```python
from build123d import *

# Parameters (mm, degrees)
ESBO_O1_W                = 700
ESBO_O1_H                = 210
RESSALTO_EXTRUS_O1_DEPTH = 2.5
RESSALTO_EXTRUS_O2_DEPTH = 150
CORTE_EXTRUS_O3_REACH    = 212
ESBO_O3_W                = 695
ESBO_O3_H                = 120
RESSALTO_EXTRUS_O5_DEPTH = 9.58
ESBO_O7_W                = 2.5
ESBO_O7_H                = 217.08
RESSALTO_EXTRUS_O6_DEPTH = 100
ESBO_O9_W                = 2.5
ESBO_O9_H                = 9.6
CORTE_EXTRUS_O4_DEPTH    = 9.5
ESBO_O10_R               = 4.5
CORTE_EXTRUS_O5_DEPTH    = 3
ESBO_O11_W               = 700
ESBO_O11_H               = 125
ESBO_O11_W_2             = 695
ESBO_O11_H_2             = 120
RESSALTO_EXTRUS_O7_DEPTH = 50
ESBO_O12_W               = 700
ESBO_O12_H               = 125
RESSALTO_EXTRUS_O8_DEPTH = 2.5


with BuildPart() as part:
    # Esboço1 → Ressalto-extrusão1 (new body)
    with BuildSketch(Plane.XY):
        Rectangle(ESBO_O1_W, ESBO_O1_H)
    extrude(amount=RESSALTO_EXTRUS_O1_DEPTH)

    # Esboço2 → Ressalto-extrusão2 (add)
    with BuildSketch(Plane.XY.offset(2.5)):
        Polygon((-347.5, 102.5), (-347.5, -105), (-350, -105), (-350, 105), (350, 105), (350, -105), (347.5, -105), (347.5, 102.5), align=None)
    extrude(amount=RESSALTO_EXTRUS_O2_DEPTH)

    # Esboço3 → Corte-extrusão3 (cut, up to next)
    with BuildSketch(Plane(origin=(0, 105, 0), x_dir=(1, 0, 0), z_dir=(0, 1, 0)), mode=Mode.PRIVATE) as corte_extrus_o3_sk1:
        with Locations((0, -62.5)):
            Rectangle(ESBO_O3_W, ESBO_O3_H)
    corte_extrus_o3_tool1 = extrude(corte_extrus_o3_sk1.sketch, amount=-CORTE_EXTRUS_O3_REACH, mode=Mode.PRIVATE) & part.part
    add(corte_extrus_o3_tool1.solids().sort_by_distance((0, 105, 62.5))[0], mode=Mode.SUBTRACT)

    # Esboço6 → Ressalto-extrusão5 (add)
    with BuildSketch(Plane.XZ.offset(105)):
        Polygon((350, 0), (350, 152.5), (347.5, 152.5), (347.5, 2.5), (-347.5, 2.5), (-347.5, 152.5), (-350, 152.5), (-350, 0), align=None)
    extrude(amount=RESSALTO_EXTRUS_O5_DEPTH)

    # Esboço7 → Ressalto-extrusão6 (add)
    with BuildSketch(Plane.ZY.offset(-347.5)):
        with Locations((151.25, -6.04)):
            Rectangle(ESBO_O7_W, ESBO_O7_H)
    ressalto_extrus_o6 = extrude(amount=RESSALTO_EXTRUS_O6_DEPTH)

    # Espelhar1: Ressalto-extrusão6 across plane
    add(ressalto_extrus_o6.mirror(Plane(origin=(0, 0, 0), x_dir=(0, 0, 1), z_dir=(1, 0, 0))))

    # Esboço9 → Corte-extrusão4 (cut)
    with BuildSketch(Plane.XY.offset(152.5)):
        with Locations((-248.75, -109.78)):
            Rectangle(ESBO_O9_W, ESBO_O9_H)
        with Locations((248.75, -109.78)):
            Rectangle(ESBO_O9_W, ESBO_O9_H)
    extrude(amount=-CORTE_EXTRUS_O4_DEPTH, mode=Mode.SUBTRACT)

    # Esboço10 → Corte-extrusão5 (cut)
    with BuildSketch(Plane(origin=(0, 105, 0), x_dir=(1, 0, 0), z_dir=(0, 1, 0))):
        with Locations((-230, -142.29)):
            Circle(ESBO_O10_R)
        with Locations((-115, -142.29)):
            Circle(ESBO_O10_R)
        with Locations((0, -142.29)):
            Circle(ESBO_O10_R)
        with Locations((115, -142.29)):
            Circle(ESBO_O10_R)
        with Locations((230, -142.29)):
            Circle(ESBO_O10_R)
    extrude(amount=-CORTE_EXTRUS_O5_DEPTH, mode=Mode.SUBTRACT)

    # Esboço11 → Ressalto-extrusão7 (add)
    with BuildSketch(Plane(origin=(0, 105, 0), x_dir=(1, 0, 0), z_dir=(0, 1, 0))):
        with Locations((0, -62.5)):
            Rectangle(ESBO_O11_W, ESBO_O11_H)
        with Locations((0, -62.5)):
            Rectangle(ESBO_O11_W_2, ESBO_O11_H_2, mode=Mode.SUBTRACT)
    extrude(amount=RESSALTO_EXTRUS_O7_DEPTH)

    # Esboço12 → Ressalto-extrusão8 (add)
    with BuildSketch(Plane(origin=(0, 155, 0), x_dir=(1, 0, 0), z_dir=(0, 1, 0))):
        with Locations((0, -62.5)):
            Rectangle(ESBO_O12_W, ESBO_O12_H)
    extrude(amount=RESSALTO_EXTRUS_O8_DEPTH)


solid = part.part
```
Can you work these out from the model? Positions are in its coordinate system, mm. A direction names the side the tool comes from. Coordinates: 2 decimals unless noted, no trailing zeros. Write each loop counter-clockwise with the first axis right and the second up, starting at its lowest first coordinate (ties: lowest second). Pieces come first, ordered by that corner, then holes. Notation, with made-up numbers: M 26.5,-9.75 L 52.5,-9.75 A17 ccw 52.5,16.25 Z; hole C 40,56.5 d6. An arc over 180 degrees is marked long. Write item = value, one per line. Start each with the question number.
Q1. Thinking about a two-plate mould opening in Z: for faces 4 (the face through (5, 102.5, 137)), 5 (the face through (-5, 20, 0)), 6 (the face through (-5, 157.5, 62)), which applies, released by +Z, released by -Z, zero draft, split by the parting line, or undercut?
Q2. If we section it at B-B, the plane x = -178: Write out the boundary of the cut face in (y, z), then the cut area to 3 significant figures.
Q3. If we section it at D-D, the plane z = 35.5: Write out the boundary of the cut face in (x, y).
Q4. If we section it at C-C, the plane y = -52: Write out the boundary of the cut face in (x, z).
Q5. If we section it at A-A, the plane y = 112.5: Write out the boundary of the cut face in (x, z), then the cut area to 3 significant figures.
Q6. I'm going to push flat-ended pins straight in: pin 1 (14.5 mm diameter, centred on x = 0, z = 142.29, fed in from -Y); pin 2 (4 mm diameter, centred on x = 81.5, z = 107, fed in from -Y); pin 3 (8 mm diameter, centred on x = 230, z = 142.29, fed in from -Y); pin 4 (10 mm diameter, centred on x = 234.5, y = -66.5, fed in from +Z). Where does each tip first touch, or does it pass through?
Q7. On a 3-axis mill with a long thin cutter (end or side, diameter ignored), from which of +Z, -Z, +X, -X, +Y, -Y can I reach the whole of each face in a straight line? I mean faces 1 (the face through (-350, 20, 77)), 2 (the face through (-5, 128, 122.5)), 3 (the face through (-5, 131, 125)). Say none if no direction works.
Q8. If I drill on L1, parallel to X at y = 104.25, z = 142.29; L2, parallel to Z at x = 0, y = 103; L3, parallel to X at y = 61, z = 133.5, over which ranges is the centre line in solid material (lowest first)? Write a range as [from, to].
Check sheet entries:
q1.face_4 = undercut
q1.face_5 = released by -Z
q1.face_6 = zero draft
q2.outline = M -114.58,0 L 157.5,0 L 157.5,125 L 105,125 L 105,152.5 L 102.5,152.5 L 102.5,122.5 L 155,122.5 L 155,2.5 L -114.58,2.5 Z
q2.area = 1,190 mm²
q3.outline = M -350,-114.58 L -347.5,-114.58 L -347.5,155 L 347.5,155 L 347.5,-114.58 L 350,-114.58 L 350,157.5 L -350,157.5 Z
q4.outline = M -350,0 L 350,0 L 350,152.5 L 247.5,152.5 L 247.5,150 L 347.5,150 L 347.5,2.5 L -347.5,2.5 L -347.5,150 L -247.5,150 L -247.5,152.5 L -350,152.5 Z
q5.outline = M -350,0 L 350,0 L 350,125 L -350,125 Z; hole M -347.5,2.5 L 347.5,2.5 L 347.5,122.5 L -347.5,122.5 Z
q5.area = 4,100 mm²
q6.pin_1 = 102.5
q6.pin_2 = 155
q6.pin_3 = through
q6.pin_4 = 2.5
q7.face_1 = +Z, -Z, -X, +Y, -Y
q7.face_2 = -Y
q7.face_3 = +Z, +X, -X, +Y
q8.L1 = [-350, -234.5], [-225.5, -119.5], [-110.5, -4.5], [4.5, 110.5], [119.5, 225.5], [234.5, 350]
q8.L2 = [0, 2.5], [122.5, 137.79], [146.79, 152.5]
q8.L3 = [-350, -347.5], [347.5, 350]
